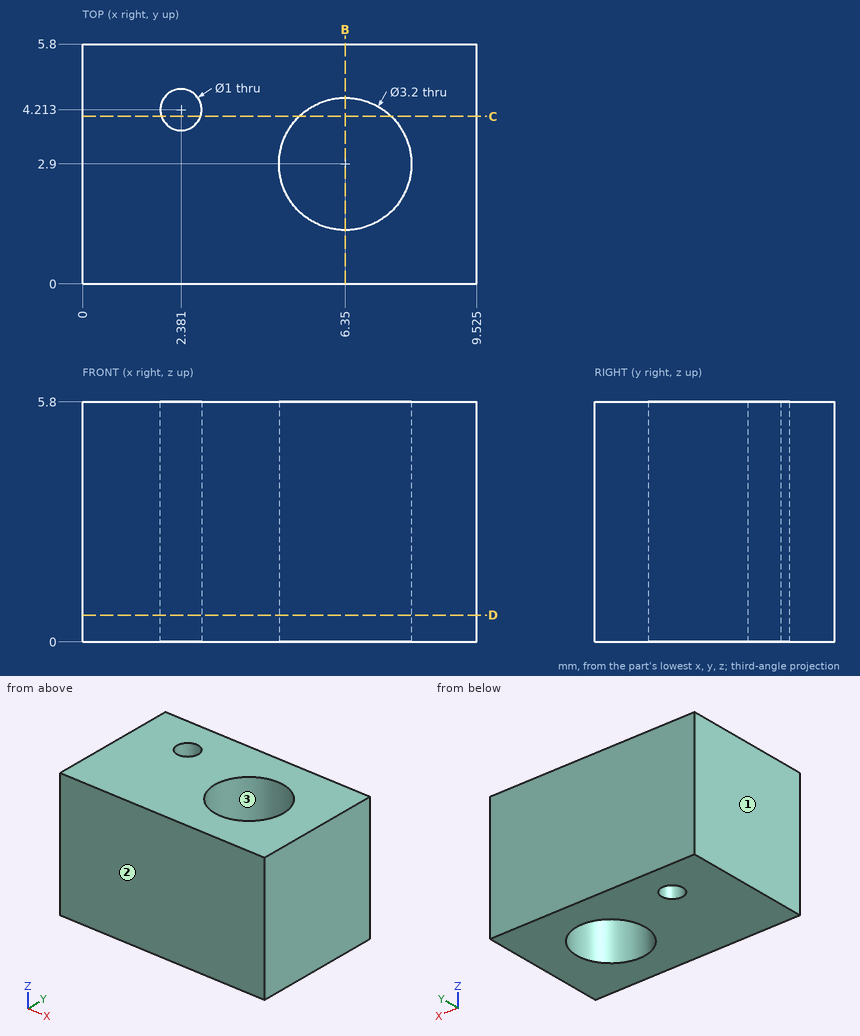
Job drawing, mm, ordinate dimensions from the low corner. One solid piece. Round coordinates to 2 decimals unless told otherwise and drop trailing zeros. Order: outer loops, then holes, each group sorted by start corner. A loop starts at its lowest first (then second) coordinate and runs counter-clockwise, first axis right, second up. Notation, with made-up numbers: (-4.5, 22.25) -> (10.5, 22.25) arc R14 ccw to (10.5, 45.25) -> close; hole circle Ø9 at (70, -9). An arc over 180 degrees is marked (long way). Answer in a Markdown table with one row per item.
1) Pin check, flat tip, straight feed: P1, Ø2, axis at x = 5, z = 0.5, coming from the -Y side. Stop position of the tip, or through.
Values:
| item | result |
|---|---|
| P1 | y = 0 |
2) Mould opens along Y. For the marked faces 1, 2 and 3 say: released by +Y, released by -Y, zero draft, split by the parting line, or undercut.
Values:
| item | result |
|---|---|
| face 1 | zero draft |
| face 2 | released by -Y |
| face 3 | undercut |
3) Band-saw the part on D-D on z = 0.65. Give the number of separate pieces and of enclosed holes in the cut face.
Values:
| item | result |
|---|---|
| separate pieces | 1 |
| enclosed holes | 2 |
4) Band-saw the part on C-C on y = 4.05. Give the cut face in (x, z) (1 decimal).
Values:
| item | result |
|---|---|
| outline | (0, 0) -> (1.9, 0) -> (1.9, 5.8) -> (0, 5.8) -> close; (2.9, 0) -> (5.2, 0) -> (5.2, 5.8) -> (2.9, 5.8) -> close; (7.5, 0) -> (9.5, 0) -> (9.5, 5.8) -> (7.5, 5.8) -> close |
5) Wall check: L1, parallel to Y at x = 6.35, z = 3.8; L2, parallel to X at y = 2.8, z = 1.3 (1 decimal); L3, parallel to Y at x = 5, z = 2.05 (1 decimal). Give the ranges that are in metal, low to high.
Values:
| item | result |
|---|---|
| L1 | 0 to 1.3, 4.5 to 5.8 |
| L2 | 0 to 4.8, 7.9 to 9.5 |
| L3 | 0 to 2, 3.8 to 5.8 |
6) Band-saw the part on B-B on x = 6.35. Give the cut face in (y, z), and give its area (3 significant figures).
Values:
| item | result |
|---|---|
| outline | (0, 0) -> (1.3, 0) -> (1.3, 5.8) -> (0, 5.8) -> close; (4.5, 0) -> (5.8, 0) -> (5.8, 5.8) -> (4.5, 5.8) -> close |
| area | 15.1 mm2 |
